Build history of the part. All positions in model axes, mm. Coordinates: 2 decimals unless noted, no trailing zeros. Order: outer loops, then holes, each group sorted by start corner. A loop starts at its lowest first (then second) coordinate and runs counter-clockwise, first axis right, second up. Notation, with made-up numbers: (63, 42.5) -> (94, 42.5) arc R21 ccw to (94, 57.5) -> close; hole circle Ø9 at (39.25, 11.5). An arc over 180 degrees is marked (long way). Write each question's results on one line, items separated by ' | '.
from build123d import *

# Parameters (mm, degrees)
BOSS_EXTRUDE1_DEPTH = 3.416
SKETCH3_R           = 2.1
CUT_EXTRUDE1_DEPTH  = 4
CHAMFER1_SIZE       = 3


with BuildPart() as part:
    # Sketch1 → Boss-Extrude1 (new body)
    with BuildSketch(Plane(origin=(0, 0, 0), x_dir=(1, 0, 0), z_dir=(0, 1, 0))):
        Polygon((0, 0), (0, 80), (20, 80), (80, 20), (80, 0), align=None)
    extrude(amount=BOSS_EXTRUDE1_DEPTH)

    # Sketch3 → Cut-Extrude1 (cut)
    with BuildSketch(Plane(origin=(0, 3.416, 0), x_dir=(1, 0, 0), z_dir=(0, 1, 0))):
        with Locations((10, 10)):
            Circle(SKETCH3_R)
        with Locations((40, 10)):
            Circle(SKETCH3_R)
        with Locations((70, 10)):
            Circle(SKETCH3_R)
        with Locations((10, 40)):
            Circle(SKETCH3_R)
        with Locations((10, 70)):
            Circle(SKETCH3_R)
    extrude(amount=-CUT_EXTRUDE1_DEPTH, mode=Mode.SUBTRACT)

    # Chamfer1
    chamfer1_edges = [part.edges().sort_by_distance(p)[0] for p in [
        (7.9, 3.416, -70),
        (7.9, 3.416, -40),
        (67.9, 3.416, -10),
        (7.9, 3.416, -10),
        (37.9, 3.416, -10),
    ]]
    chamfer(chamfer1_edges, length=CHAMFER1_SIZE)


solid = part.part
Item 1: Slice it at D-D, the plane y = 2.6. List the corners of the cut face in (x, z).
Answer:
outline: (0, -80) -> (20, -80) -> (80, -20) -> (80, 0) -> (0, 0) -> close; hole circle Ø8.57 at (10, -70); hole circle Ø8.57 at (10, -40); hole circle Ø8.57 at (10, -10); hole circle Ø8.57 at (40, -10); hole circle Ø8.57 at (70, -10)
Item 2: Pin check, flat tips, straight feed: pin 1 (1.5 mm diameter, centred on x = 65.5, y = 0.5, fed in from -Z); pin 2 (5 mm diameter, centred on x = 10, z = -70, fed in from +Y); pin 3 (3.5 mm diameter, centred on x = 10, z = -10, fed in from -Y); pin 4 (5.5 mm diameter, centred on x = 40, z = -10, fed in from +Y). Stop position of each tip, or through.
Answer:
pin 1: stops at z = -35.25 | pin 2: stops at y = 0.82 | pin 3: passes through | pin 4: stops at y = 1.07
Item 3: Pull direction X, two halves, no side cores. Call faces 1 (the cylindrical face through (71.13, 0.21, -11.77)), 2 (the flat face through (10, 2, -80)), 3 (the flat face through (50, 2, -50)), 4 (the cylindrical face through (8.334, 0.211, -38.722)): released by +X, released by -X, zero draft, split by the parting line, or undercut.
Answer:
face 1: undercut | face 2: zero draft | face 3: released by +X | face 4: undercut
Item 4: Drill centre lines: line 1 (X direction, y = 0.15, z = -10); line 2 (Z direction, x = 10, y = 0.1); line 3 (Z direction, x = 9.5, y = 2.4). Where is each one in solid material? Low to high. Write a range as from..to.
Answer:
line 1: x = 0..7.9, 12.1..37.9, 42.1..67.9, 72.1..80 | line 2: z = -80..-72.1, -67.9..-42.1, -37.9..-12.1, -7.9..0 | line 3: z = -80..-74.05, -65.95..-44.05, -35.95..-14.05, -5.95..0
Item 5: Slice it at C-C, the plane z = -10. List the corners of the cut face in (x, y), and give its area (3 significant figures).
Answer:
outline: (0, 0) -> (7.9, 0) -> (7.9, 0.42) -> (4.9, 3.42) -> (0, 3.42) -> close; (12.1, 0) -> (37.9, 0) -> (37.9, 0.42) -> (34.9, 3.42) -> (15.1, 3.42) -> (12.1, 0.42) -> close; (42.1, 0) -> (67.9, 0) -> (67.9, 0.42) -> (64.9, 3.42) -> (45.1, 3.42) -> (42.1, 0.42) -> close; (72.1, 0) -> (80, 0) -> (80, 3.42) -> (75.1, 3.42) -> (72.1, 0.42) -> close | area: 203 mm^2
Item 6: Slice it at B-B, the plane x = 40. List the corners of the cut face in (y, z), and give its area (3 significant figures).
Answer:
outline: (0, -60) -> (3.42, -60) -> (3.42, -15.1) -> (0.42, -12.1) -> (0, -12.1) -> close; (0, -7.9) -> (0.42, -7.9) -> (3.42, -4.9) -> (3.42, 0) -> (0, 0) -> close | area: 182 mm^2
Item 7: Slice it at A-A, the plane x = 10. List the corners of the cut face in (y, z).
Answer:
outline: (0, -80) -> (3.42, -80) -> (3.42, -75.1) -> (0.42, -72.1) -> (0, -72.1) -> close; (0, -67.9) -> (0.42, -67.9) -> (3.42, -64.9) -> (3.42, -45.1) -> (0.42, -42.1) -> (0, -42.1) -> close; (0, -37.9) -> (0.42, -37.9) -> (3.42, -34.9) -> (3.42, -15.1) -> (0.42, -12.1) -> (0, -12.1) -> close; (0, -7.9) -> (0.42, -7.9) -> (3.42, -4.9) -> (3.42, 0) -> (0, 0) -> close
